Design review of the part built by this model. Coordinates are the model's own, in mm. Face numbers are marked on the shaded views. A direction names the side the tool comes from. Give positions to 0.01 mm unless a question says otherwise; leave off trailing zeros. Loops run counter-clockwise (first coordinate to the right, second up) from the corner with the lowest first, then second, coordinate; pieces in that order, holes last.
from build123d import *

# Parameters (mm, degrees)
BOSS_EXTRUDE1_DEPTH    = 15
BOSS_EXTRUDE2_DEPTH    = 10
SKETCH3_R              = 3.25
CUT_EXTRUDE1_DEPTH     = 9
CUT_EXTRUDE2_START     = -7
SKETCH4_R              = 6
CUT_EXTRUDE2_DEPTH     = 7
CHAMFER1_START         = 3
CHAMFER1_2_DEPTH       = 7
CHAMFER1_3_OUTLINE_R   = 12
CHAMFER1_3_OUTLINE_R_2 = 6
CHAMFER1_3_DEPTH       = 7
CHAMFER2_SIZE          = 5
CHAMFER2_SIZE2         = 3


with BuildPart() as part:
    # Sketch1 → Boss-Extrude1 (new body)
    with BuildSketch(Plane(origin=(0, 0, 0), x_dir=(1, 0, 0), z_dir=(0, 1, 0))):
        with BuildLine():
            Line((-30, -388.070415552), (30, -388.070415552))
            Line((30, -388.070415552), (30, -372.350901436))
            ThreePointArc((30, -372.350901436), (0, -375.726435625), (-30, -372.350901436))
            Line((-30, -372.350901436), (-30, -388.070415552))
        make_face()
        with BuildLine():
            Line((-21, -382.710658494), (-21, -377.710658494))
            ThreePointArc((-21, -377.710658494), (-23, -375.710658494), (-25, -377.710658494))
            Line((-25, -377.710658494), (-25, -382.710658494))
            ThreePointArc((-25, -382.710658494), (-23, -384.710658494), (-21, -382.710658494))
        make_face(mode=Mode.SUBTRACT)
        with BuildLine():
            Line((25, -377.710658494), (25, -382.710658494))
            ThreePointArc((25, -382.710658494), (23, -384.710658494), (21, -382.710658494))
            Line((21, -382.710658494), (21, -377.710658494))
            ThreePointArc((21, -377.710658494), (23, -375.710658494), (25, -377.710658494))
        make_face(mode=Mode.SUBTRACT)
    extrude(amount=BOSS_EXTRUDE1_DEPTH)

    # Sketch2 → Boss-Extrude2 (add)
    with BuildSketch(Plane(origin=(0, 0, 0), x_dir=(1, 0, 0), z_dir=(0, 1, 0))):
        with BuildLine():
            Line((30, -372.350901436), (19.377517729, -330.775495649))
            ThreePointArc((19.377517729, -330.775495649), (0, -315.726435625), (-19.377517729, -330.775495649))
            Line((-19.377517729, -330.775495649), (-30, -372.350901436))
            ThreePointArc((-30, -372.350901436), (0, -375.726435625), (30, -372.350901436))
        make_face()
    extrude(amount=BOSS_EXTRUDE2_DEPTH)

    # Sketch3 → Cut-Extrude1 (cut)
    with BuildSketch(Plane(origin=(0, 10, 0), x_dir=(1, 0, 0), z_dir=(0, 1, 0))):
        with Locations(Location((0, -335.726435625, 0), (0, 0, 270))):
            Circle(SKETCH3_R)
    extrude(amount=-CUT_EXTRUDE1_DEPTH, mode=Mode.SUBTRACT)

    # Sketch4 → Cut-Extrude2 (cut)
    with BuildSketch(Plane(origin=(0, 10, 0), x_dir=(1, 0, 0), z_dir=(0, 1, 0)).offset(CUT_EXTRUDE2_START)):
        with BuildLine():
            Line((30, -372.350901436), (19.377517729, -330.775495649))
            ThreePointArc((19.377517729, -330.775495649), (0, -315.726435625), (-19.377517729, -330.775495649))
            Line((-19.377517729, -330.775495649), (-30, -372.350901436))
            ThreePointArc((-30, -372.350901436), (0, -375.726435625), (30, -372.350901436))
        make_face()
        with Locations(Location((0, -335.726435625, 0), (0, 0, 270))):
            Circle(SKETCH4_R, mode=Mode.SUBTRACT)
    extrude(amount=CUT_EXTRUDE2_DEPTH, mode=Mode.SUBTRACT)

    # Chamfer1: read off the stored shape, not the designer's step
    # Chamfer1 outline → Chamfer1 (revolve)
    with BuildSketch(Plane.XY.offset(335.726435625)):
        Polygon((26, 3), (12, 10), (12, 3), align=None)
    revolve(axis=Axis((0, 0, 335.726435625), (0, 1, 0)))

    # Chamfer1 2 outline → Chamfer1 2 (cut)
    with BuildSketch(Plane(origin=(0, 0, 0), x_dir=(1, 0, 0), z_dir=(0, 1, 0)).offset(CHAMFER1_START)):
        with BuildLine():
            ThreePointArc((-19.377517729, -330.775495649), (0, -315.726435625), (19.377517729, -330.775495649))
            Line((19.377517729, -330.775495649), (24.033863727, -349))
            Line((24.033863727, -349), (27, -349))
            Line((27, -349), (27, -308))
            Line((27, -308), (-27, -308))
            Line((-27, -308), (-27, -349))
            Line((-27, -349), (-24.033863727, -349))
            Line((-24.033863727, -349), (-19.377517729, -330.775495649))
        make_face()
    extrude(amount=CHAMFER1_2_DEPTH, mode=Mode.SUBTRACT)

    # Chamfer1 3 outline → Chamfer1 3 (add)
    with BuildSketch(Plane(origin=(0, 0, 0), x_dir=(1, 0, 0), z_dir=(0, 1, 0)).offset(CHAMFER1_START)):
        with Locations((0, -335.726435625)):
            Circle(CHAMFER1_3_OUTLINE_R)
        with Locations((0, -335.726435625)):
            Circle(CHAMFER1_3_OUTLINE_R_2, mode=Mode.SUBTRACT)
    extrude(amount=CHAMFER1_3_DEPTH)

    # Chamfer2
    chamfer2_edges = [part.edges().sort_by_distance(p)[0] for p in [
        (0, 10, 332.476435625),
    ]]
    chamfer2_side = [part.faces().sort_by_distance(p)[0] for p in [
        (-11.660588745, 10, 335.726435625),
    ]]
    chamfer(chamfer2_edges, length=CHAMFER2_SIZE, length2=CHAMFER2_SIZE2, reference=chamfer2_side[0])


solid = part.part
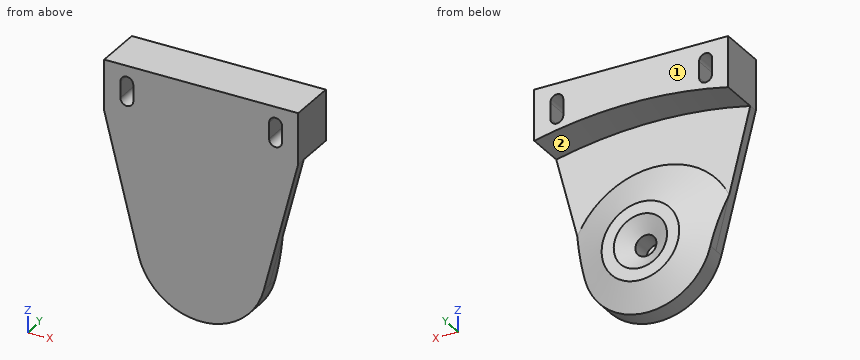
Q1. Tool access review of the marked faces 1 and 2: name each direction out of +Z, -Z, +X, -X, +Y, -Y from which nothing blocks a thin tool from reaching the whole face with its end or side.
Results:
face 1: +Z, -Z, +X, -X, +Y
face 2: +Y
Q2. Take a section at C-C (x = 0). Give the boundary of the cut face in (y, z).
Results:
outline: (0, 315.73) - (6, 315.73) - (10, 323.73) - (10, 327.48) - (7, 332.48) - (1, 332.48) - (1, 338.98) - (7, 338.98) - (10, 343.98) - (10, 347.73) - (3, 361.73) - (3, 375.73) - (15, 375.73) - (15, 388.07) - (0, 388.07) - close
Q3. Take a section at B-B (y = 2). Give the boundary of the cut face in (x, z), plus the area to 3 significant figures.
Results:
outline: (-30, 372.35) - (-19.38, 330.78) arc R20 ccw to (19.38, 330.78) - (30, 372.35) - (30, 388.07) - (-30, 388.07) - close; hole (-25, 377.71) arc R2 ccw to (-21, 377.71) - (-21, 382.71) arc R2 ccw to (-25, 382.71) - close; hole circle Ø6.5 at (0, 335.73); hole (21, 377.71) arc R2 ccw to (25, 377.71) - (25, 382.71) arc R2 ccw to (21, 382.71) - close
area: 3,330 mm2
Q4. Insertion check: pin 1 (1 mm diameter, centred on x = -11, z = 348.5, fed in from +Y); pin 2 (12 mm diameter, centred on x = -3, z = 333, fed in from +Y); pin 3 (6 mm diameter, centred on y = 6, z = 326, fed in from +X). Each pin has a flat end and moves straight along its axis. Give the tip position at first contact, or say it passes through.
Results:
pin 1: stops at y = 7.82
pin 2: stops at y = 10
pin 3: stops at x = 18.83
Q5. Wall thickness on line 1 (X direction, y = 4.5, z = 377.5); line 2 (Y direction, x = 21, z = 357); line 3 (Z direction, x = 2.5, y = 11.25): over which ranges is each line inside the solid? List them lowest first.
Results:
line 1: x = -30 to -24.99, -21.01 to 21.01, 24.99 to 30
line 2: y = 0 to 3
line 3: z = 375.7 to 388.07
Q6. Take a section at A-A (y = 13). Give the boundary of the cut face in (x, z), plus the area to 3 significant figures.
Results:
outline: (-30, 372.35) arc R135 cw to (30, 372.35) - (30, 388.07) - (-30, 388.07) - close; hole (-25, 377.71) arc R2 ccw to (-21, 377.71) - (-21, 382.71) arc R2 ccw to (-25, 382.71) - close; hole (21, 377.71) arc R2 ccw to (25, 377.71) - (25, 382.71) arc R2 ccw to (21, 382.71) - close
area: 743 mm2
